```python
from build123d import *

# Parameters (mm, degrees)
MAIN_DEPTH         = 90
SKETCH2_R          = 5
PLOT_DEPTH         = 2.5
SKETCH3_R          = 1.25
HOLEFIX_DEPTH      = 14
SKETCH4_R          = 1.25
CUT_EXTRUDE4_DEPTH = 14
SKETCH5_W          = 31.518406853
SKETCH5_H          = 19.182170192
CUT_EXTRUDE5_DEPTH = 91


with BuildPart() as part:
    # Sketch1 → Main (new body)
    with BuildSketch(Plane.XY):
        Polygon((-10, 7.5), (0, 7.5), (0, 3.95), (-2.5, 3.95), (-2.5, 1.05), (0, 1.05), (0, 0), (7, 0), (7, 10.5), (-10, 10.5), align=None)
    extrude(amount=MAIN_DEPTH)

    # Sketch2 → Plot (add)
    with BuildSketch(Plane(origin=(0, 10.5, 0), x_dir=(1, 0, 0), z_dir=(0, 1, 0))):
        with Locations((-5.6, -85)):
            Circle(SKETCH2_R)
        with Locations((-5.6, -10.2)):
            Circle(SKETCH2_R)
    extrude(amount=PLOT_DEPTH)

    # Sketch3 → HoleFix (cut, through all)
    with BuildSketch(Plane(origin=(0, 13, 0), x_dir=(1, 0, 0), z_dir=(0, 1, 0))):
        with Locations((-5.6, -10.2)):
            Circle(SKETCH3_R)
        with Locations((-5.6, -85)):
            Circle(SKETCH3_R)
    extrude(amount=-HOLEFIX_DEPTH, mode=Mode.SUBTRACT)

    # Sketch4 → Cut-Extrude4 (cut, through all)
    with BuildSketch(Plane(origin=(7, 0, 0), x_dir=(0, 0, -1), z_dir=(0, 1, 0))):
        with Locations((-85, 3.5)):
            Circle(SKETCH4_R)
        with Locations((-5, 3.5)):
            Circle(SKETCH4_R)
    extrude(amount=CUT_EXTRUDE4_DEPTH, mode=Mode.SUBTRACT)


with BuildPart() as body_2:
    # Mirror2: mirrored copy
    add(part.part.mirror(Plane.ZX.offset(18.5)))


with BuildPart() as part_1:
    add(part.part)

    # Sketch5 → Cut-Extrude5 (cut, through all)
    with BuildSketch(Plane.XY.offset(90)):
        with Locations((-2.991193443, 6.5365617)):
            Rectangle(SKETCH5_W, SKETCH5_H)
    extrude(amount=-CUT_EXTRUDE5_DEPTH, mode=Mode.SUBTRACT)


solid = body_2.part
```
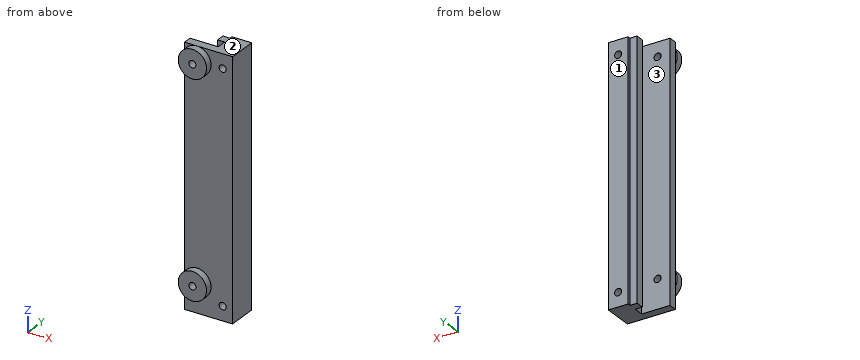
Work out the finished part from the listing and answer in its coordinate system (mm). Face numbers are marked on the shaded views. Round coordinates to 2 decimals unless told otherwise and drop trailing zeros. Write each loop counter-clockwise with the first axis right and the second up, starting at its lowest first coordinate (ties: lowest second). Pieces come first, ordered by that corner, then holes. Notation, with made-up numbers: (-10, -32) -> (6, -32) arc R26 cw to (6, -10) -> close; hole circle Ø2 at (32, 68). An arc over 180 degrees is marked (long way). Write each question's results on one line, items separated by ' | '.
1) The part is cut by section C-C (y = 25.5). Write down the section's boundary in (x, z).
Findings:
outline: circle Ø10 at (-5.6, 10.2); circle Ø10 at (-5.6, 85); hole circle Ø2.5 at (-5.6, 10.2); hole circle Ø2.5 at (-5.6, 85)
2) The part is cut by section D-D (z = 10.2). Write down the section's boundary in (x, y), and give its area (3 significant figures).
Findings:
outline: (-10.6, 24) -> (-6.85, 24) -> (-6.85, 29.5) -> (-10, 29.5) -> (-10, 26.5) -> (-10.6, 26.5) -> close; (-4.35, 24) -> (-0.6, 24) -> (-0.6, 26.5) -> (7, 26.5) -> (7, 37) -> (0, 37) -> (0, 35.95) -> (-2.5, 35.95) -> (-2.5, 33.05) -> (0, 33.05) -> (0, 29.5) -> (-4.35, 29.5) -> close | area: 122 mm²
3) Consider line 1 along Z through (x, y) = (3.5, 32.25); line 2 along Z through (x, y) = (-5.6, 26.95); line 3 along Z through (x, y) = (-5.6, 25.2). Determine where each line is inside the solid, lowest interval first. Write a range as [from, to].
Findings:
line 1: z = [0, 3.75], [6.25, 83.75], [86.25, 90] | line 2: z = [0, 8.95], [11.45, 83.75], [86.25, 90] | line 3: z = [5.2, 8.95], [11.45, 15.2], [80, 83.75], [86.25, 90]
4) The part is cut by section B-B (x = 3.5). Write down the section's boundary in (y, z), and give its area (4 significant figures).
Findings:
outline: (26.5, 0) -> (37, 0) -> (37, 3.75) -> (26.5, 3.75) -> close; (26.5, 6.25) -> (37, 6.25) -> (37, 83.75) -> (26.5, 83.75) -> close; (26.5, 86.25) -> (37, 86.25) -> (37, 90) -> (26.5, 90) -> close | area: 892.5 mm²
5) Flat-ended cylindrical pins translate along their axes: pin 1 (1.5 mm diameter, centred on x = 1.5, z = 33.5, fed in from -Y); pin 2 (2 mm diameter, centred on x = 3.5, z = 5, fed in from -Y); pin 3 (1.5 mm diameter, centred on y = 27.5, z = 58, fed in from -X); pin 4 (2 mm diameter, centred on x = -5.5, y = 28.5, fed in from -Z). Find the tip coordinate at first contact, or state that the pin passes through.
Findings:
pin 1: stops at y = 26.5 | pin 2: passes through | pin 3: stops at x = -10 | pin 4: stops at z = 0
6) The part is cut by section A-A (z = 85). Write down the section's boundary in (x, y).
Findings:
outline: (-10.6, 24) -> (-6.85, 24) -> (-6.85, 29.5) -> (-10, 29.5) -> (-10, 26.5) -> (-10.6, 26.5) -> close; (-4.35, 24) -> (-0.6, 24) -> (-0.6, 26.5) -> (2.25, 26.5) -> (2.25, 37) -> (0, 37) -> (0, 35.95) -> (-2.5, 35.95) -> (-2.5, 33.05) -> (0, 33.05) -> (0, 29.5) -> (-4.35, 29.5) -> close; (4.75, 26.5) -> (7, 26.5) -> (7, 37) -> (4.75, 37) -> close
7) For a pull along Y with two mould halves and no side action, classify the marked faces 1, 2 and 3 as +Y half, -Y half, draft (parallel to the pull), parting line (faces both ways), or undercut.
Findings:
face 1: +Y half | face 2: draft | face 3: undercut
